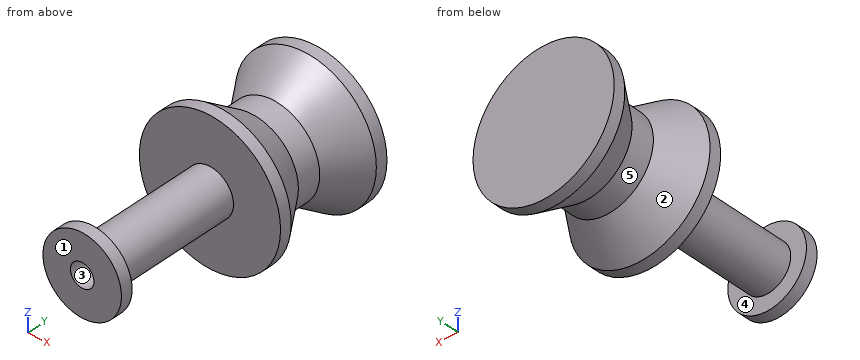
from build123d import *

# Parameters (mm, degrees)
F0_R      = 2
F0_R_2    = 1
F1_DEPTH  = 22
F0_R_3    = 6
F0_R_4    = 3.5
F2_DEPTH  = 1
F2_FACE_R = 6
F3_DEPTH  = 3
F3_TAPER  = 35
F4_DEPTH  = 2
F7_R      = 3.33782825
F7_R_2    = 2
F7_R_3    = 1
F8_DEPTH  = 1


# Not quite as in the source:
# - a feature of the source that left no trace in its solid (it failed there, or was rolled back) is left out
# - a pattern or mirror of a feature is missing from the dataset's text; its kind, count and spacing are read off the source's solid


with BuildPart() as f1:
    # F0 (on Front) → F1 (new body)
    with BuildSketch(Plane.XZ):
        Circle(F0_R)
        Circle(F0_R_2, mode=Mode.SUBTRACT)
    extrude(amount=F1_DEPTH)

    # F2_copies: F2 across plane


with BuildPart() as f2:
    # F0 (on Front) → F2 (new body)
    with BuildSketch(Plane.XZ):
        Circle(F0_R_3)
        Circle(F0_R_4, mode=Mode.SUBTRACT)
        Circle(F0_R_4)
        Circle(F0_R, mode=Mode.SUBTRACT)
        Circle(F0_R)
        Circle(F0_R_2, mode=Mode.SUBTRACT)
        Circle(F0_R_2)
    extrude(amount=F2_DEPTH)


with BuildPart() as f1_1:
    add(f1.part)
    add(f2.part.mirror(Plane(origin=(0, -5, 0), x_dir=(0, 0, -1), z_dir=(0, -1, 0))))


    add(f2.part)  # F3 merges F2
    # F2_face (on face) → F3 (join)
    with BuildSketch(Plane.XZ.offset(1)):
        Circle(F2_FACE_R)
    f3 = extrude(amount=F3_DEPTH, taper=F3_TAPER)

    # F3_copies: F3 across plane
    add(f3.mirror(Plane(origin=(0, -5, 0), x_dir=(0, 0, -1), z_dir=(0, -1, 0))))

    # F4 (add): faces of the model
    f4_faces = [f1_1.faces().sort_by_distance(p)[0] for p in [
        (-3.7890863377, -4, 0),
        (0, -4, 0),
    ]]
    extrude(f4_faces, amount=F4_DEPTH)

    # F7 (on face) → F8 (join)
    with BuildSketch(Plane.XZ.offset(22)):
        Circle(F7_R)
        Circle(F7_R_2, mode=Mode.SUBTRACT)
        Circle(F7_R_2)
        Circle(F7_R_3, mode=Mode.SUBTRACT)
    extrude(amount=-F8_DEPTH)


solid = f1_1.part
Work out the finished part from the listing and answer in its coordinate system (mm). Face numbers are marked on the shaded views. A direction names the side the tool comes from. Give positions to 0.01 mm unless a question says otherwise; leave off trailing zeros. Order: outer loops, then holes, each group sorted by start corner. A loop starts at its lowest first (then second) coordinate and runs counter-clockwise, first axis right, second up. Notation, with made-up numbers: (-9.5, -31.5) -> (22.5, -31.5) arc R17 cw to (22.5, -10.5) -> close; hole circle Ø11 at (8.5, 10). An arc over 180 degrees is marked (long way). Answer as a JSON object with one key per item and string values. Group by question number.
1. Consider line 1 along X through (y, z) = (-16.25, 0); line 2 along Y through (x, z) = (0.5, 3). Determine where each line is inside the solid, lowest interval first. Write a range as [from, to].
2. A tool of negligible diameter and unlimited length cuts with its end or side. For the marked faces 1 and 2, from which of +Z, -Z, +X, -X, +Y, -Y can it reach the whole face along a straight path? Write none if from no direction.
3. Section A-A on x = 0 is taken. Determine the outline of the cut face in (y, z), plus the area to 3 significant figures.
4. The mould has two halves that part along X. Classify the marked faces 3, 4 and 5: released by +X, released by -X, zero draft, split by the parting line, or undercut.
5. Flat-ended cylindrical pins translate along their axes: pin 1 Ø1.5 at (x, y) = (3, -11) entering from +Z; pin 2 Ø2 at (x, y) = (0.5, -18.5) entering from +Z; pin 3 Ø6 at (y, z) = (-5.5, -4) entering from +X. Find the tip coordinate at first contact, or state that the pin passes through.
6. Section B-B on y = -14.75 is taken. Determine the outline of the cut face in (x, z), plus the area to 3 significant figures.
7. Section C-C on y = -1.5 is taken. Determine the outline of the cut face in (x, z), plus the area to 3 significant figures.
Result sheet:
{
 "1": {"line 1": "x = [-2, -1], [1, 2]", "line 2": "y = [-22, -21], [-10, 0]"},
 "2": {"face 1": "+Z, -Z, +X, -X, -Y", "face 2": "none"},
 "3": {"outline": "(-22, -3.34) -> (-21, -3.34) -> (-21, -2) -> (-10, -2) -> (-10, -6) -> (-9, -6) -> (-6, -3.9) -> (-4, -3.9) -> (-1, -6) -> (0, -6) -> (0, 6) -> (-1, 6) -> (-4, 3.9) -> (-6, 3.9) -> (-9, 6) -> (-10, 6) -> (-10, 2) -> (-21, 2) -> (-21, 3.34) -> (-22, 3.34) -> (-22, 1) -> (-10, 1) -> (-10, -1) -> (-22, -1) -> close", "area": "126 mm^2"},
 "4": {"face 3": "undercut", "face 4": "zero draft", "face 5": "split by the parting line"},
 "5": {"pin 1": "passes through", "pin 2": "stops at z = 2", "pin 3": "stops at x = 4.75"},
 "6": {"outline": "circle Ø4 at (0, 0); hole circle Ø2 at (0, 0)", "area": "9.42 mm^2"},
 "7": {"outline": "circle Ø11.3 at (0, 0)", "area": "100 mm^2"}
}
